Source: CAD feature listing. Evaluate the final solid. Frame: model axes, mm. Face numbers are marked on the shaded views. Give positions to 0.01 mm unless a question says otherwise; leave off trailing zeros. Write each loop counter-clockwise with the first axis right and the second up, starting at its lowest first coordinate (ties: lowest second). Pieces come first, ordered by that corner, then holes. Notation, with made-up numbers: (3, -19.5) -> (37, -19.5) arc R14 ccw to (37, -4.5) -> close; hole circle Ø6 at (88, -30). An arc over 180 degrees is marked (long way). Answer as a JSON object with one key per item and string values. Group by question number.
Item 1: First-contact query: pin 1 Ø4 at (x, y) = (13, 25) entering from -Z; pin 2 Ø10 at (y, z) = (-11, 54) entering from -X; pin 3 Ø5 at (x, z) = (-5.5, 63) entering from -Y. Flat tips, straight axial feed; report the tip coordinate or a pass-through.
Item 2: Section query D-D on y = 4. Return the cut outline in (x, z).
Item 3: Section query B-B on z = 38.1. Return the cut outline in (x, y).
Item 4: Pull-direction query (Y, two-part tool) for the marked faces 1, 2 and 3; classes: pulls with the +Y half, pulls with the -Y half, needs draft (parallel to the pull), parting line crosses it, or undercut.
Item 5: Section query C-C on y = 18. Return the cut outline in (x, z), plus the area to 3 significant figures.
Item 6: Section query A-A on x = 0. Return the cut outline in (y, z), plus the area to 3 significant figures.
from build123d import *

# Parameters (mm, degrees)
SKETCH1_R           = 16.7005
SKETCH1_R_2         = 12.7
BOSS_EXTRUDE1_DEPTH = 76.2
SKETCH2_R           = 16.764
SKETCH2_R_2         = 12.7
BOSS_EXTRUDE2_DEPTH = 38.1
SKETCH4_R           = 12.7
CUT_EXTRUDE2_DEPTH  = 77.2000001
CUT_EXTRUDE3_REACH  = 56.801
SKETCH5_R           = 12.7


with BuildPart() as part:
    # Sketch1 → Boss-Extrude1 (new body)
    with BuildSketch(Plane.XY):
        Circle(SKETCH1_R)
        Circle(SKETCH1_R_2, mode=Mode.SUBTRACT)
    extrude(amount=BOSS_EXTRUDE1_DEPTH)

    # Sketch2 → Boss-Extrude2 (add)
    with BuildSketch(Plane(origin=(0, 0, 0), x_dir=(1, 0, 0), z_dir=(0, 1, 0))):
        with Locations((0, -38.1)):
            Circle(SKETCH2_R)
        with Locations((0, -38.1)):
            Circle(SKETCH2_R_2, mode=Mode.SUBTRACT)
    extrude(amount=BOSS_EXTRUDE2_DEPTH)

    # Sketch4 → Cut-Extrude2 (cut, through all)
    with BuildSketch(Plane.XY.offset(76.2)):
        Circle(SKETCH4_R)
    extrude(amount=-CUT_EXTRUDE2_DEPTH, mode=Mode.SUBTRACT)

    # Sketch5 → Cut-Extrude3 (cut, up to next)
    with BuildSketch(Plane(origin=(0, 38.1, 0), x_dir=(1, 0, 0), z_dir=(0, 1, 0)), mode=Mode.PRIVATE) as cut_extrude3_sk1:
        with Locations((0, -38.1)):
            Circle(SKETCH5_R)
    cut_extrude3_tool1 = extrude(cut_extrude3_sk1.sketch, amount=-CUT_EXTRUDE3_REACH, mode=Mode.PRIVATE) & part.part
    add(cut_extrude3_tool1.solids().sort_by_distance((0, 38.1, 38.1))[0], mode=Mode.SUBTRACT)


solid = part.part
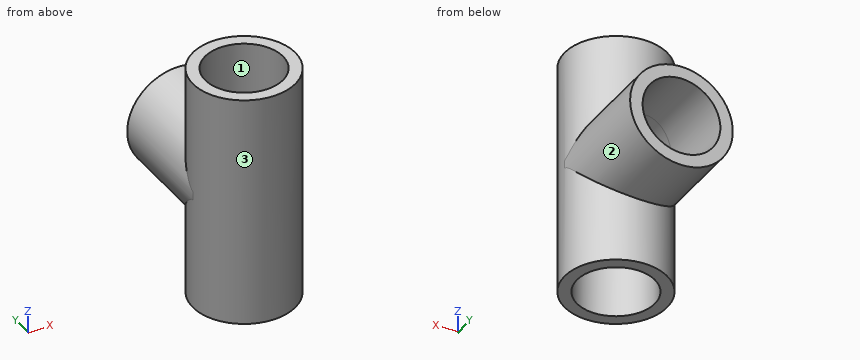
Worked answers:
{
 "1": {"pin 1": "z = 25.45", "pin 2": "x = -15.59", "pin 3": "y = -16.43"},
 "2": {"outline": "(-16.21, 0) -> (-12.05, 0) -> (-12.05, 34.1) arc R12.7 cw to (-12.05, 42.1) -> (-12.05, 76.2) -> (-16.21, 76.2) -> (-16.21, 42.36) arc R16.76 ccw to (-16.21, 33.84) -> close; (12.05, 0) -> (16.21, 0) -> (16.21, 33.84) arc R16.76 ccw to (16.21, 42.36) -> (16.21, 76.2) -> (12.05, 76.2) -> (12.05, 42.1) arc R12.7 cw to (12.05, 34.1) -> close"},
 "3": {"outline": "(-16.76, 0) -> (-16.7, 0) arc R16.7 ccw to (16.7, 0) -> (16.76, 0) -> (16.76, 38.1) -> (12.7, 38.1) -> (12.7, 0) arc R12.7 cw to (-12.7, 0) -> (-12.7, 38.1) -> (-16.76, 38.1) -> close"},
 "4": {"face 1": "undercut", "face 2": "needs draft", "face 3": "parting line crosses it"},
 "5": {"outline": "circle Ø33.53 at (0, 38.1); hole circle Ø25.4 at (0, 38.1)", "area": "376 mm^2"},
 "6": {"outline": "(-16.7, 0) -> (-12.7, 0) -> (-12.7, 76.2) -> (-16.7, 76.2) -> close; (12.7, 0) -> (16.7, 0) -> (16.7, 21.34) -> (38.1, 21.34) -> (38.1, 25.4) -> (12.7, 25.4) -> close; (12.7, 50.8) -> (38.1, 50.8) -> (38.1, 54.86) -> (16.7, 54.86) -> (16.7, 76.2) -> (12.7, 76.2) -> close", "area": "682 mm^2"}
}
